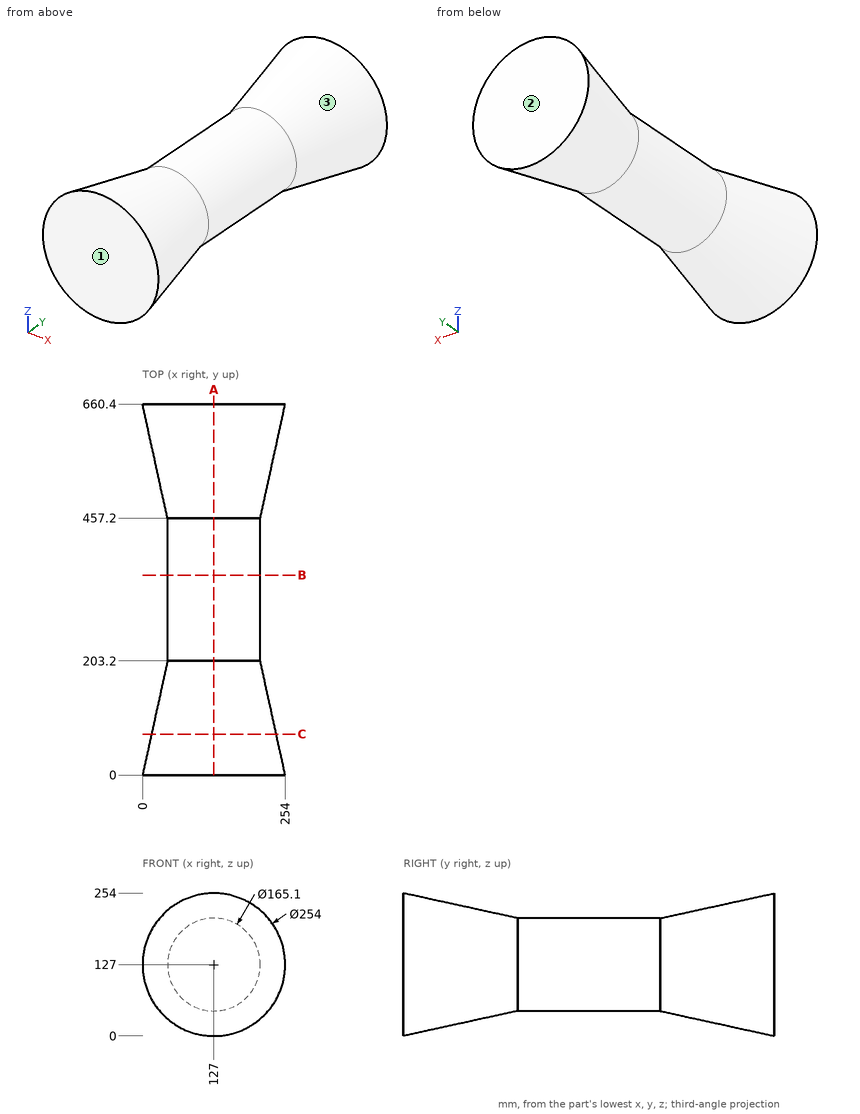
For this review, use the dimensioned drawing (mm, ordinates from the lowest corner) and the shaded views. Coordinates: 2 decimals unless noted, no trailing zeros. Order: outer loops, then holes, each group sorted by start corner. A loop starts at its lowest first (then second) coordinate and runs counter-clockwise, first axis right, second up. Notation, with made-up numbers: (67.5, 48) - (105.5, 48) arc R32 ccw to (105.5, 83) - close; hole circle Ø1 at (58, 1). An arc over 180 degrees is marked (long way). Answer as a JSON object with one key per item and string values. Group by question number.
1. We need section A-A on x = 127. State the section outline as (y, z) points, then the cut area to 3 significant figures.
2. For probe 1 along Z at (x, y) = (196.5, 490); probe 2 along X at (y, z) = (262.5, 58); probe 3 along Z at (x, y) = (76, 83.5), list the stretches that pass through material, from the lowest coordinate up.
3. We need section C-C on y = 73. State the section outline as (x, z) points, then the cut area to 3 significant figures.
4. We need section B-B on y = 356. State the section outline as (x, z) points, then the cut area to 3 significant figures.
5. The part is to be moulded in two halves that separate along Y. For the marked faces 1, 2 and 3, say which applies: pulls with the +Y half, pulls with the -Y half, needs draft (parallel to the pull), parting line crosses it, or undercut.
6. Clearance check with flat-ended pins moving along their axes: P1, Ø8, axis at x = 58, y = 341.5, coming from the +Z side; P2, Ø10, axis at x = 87.5, y = 246, coming from the +Z side (3 decimals); P3, Ø12, axis at x = 181, y = 82, coming from the +Z side. State where each tip first meets the part, or that it passes through.
Final values:
{
 "1": {"outline": "(0, 0) - (203.2, 44.45) - (457.2, 44.45) - (660.4, 0) - (660.4, 254) - (457.2, 209.55) - (203.2, 209.55) - (0, 254) - close", "area": "127,000 mm²"},
 "2": {"probe 1": "70.25 to 183.75", "probe 2": "81.68 to 172.32", "probe 3": "30.97 to 223.03"},
 "3": {"outline": "circle Ø222.06 at (127, 127)", "area": "38,700 mm²"},
 "4": {"outline": "circle Ø165.1 at (127, 127)", "area": "21,400 mm²"},
 "5": {"face 1": "pulls with the -Y half", "face 2": "pulls with the +Y half", "face 3": "undercut"},
 "6": {"P1": "z = 177.89", "P2": "z = 201.995", "P3": "z = 225.27"}
}
